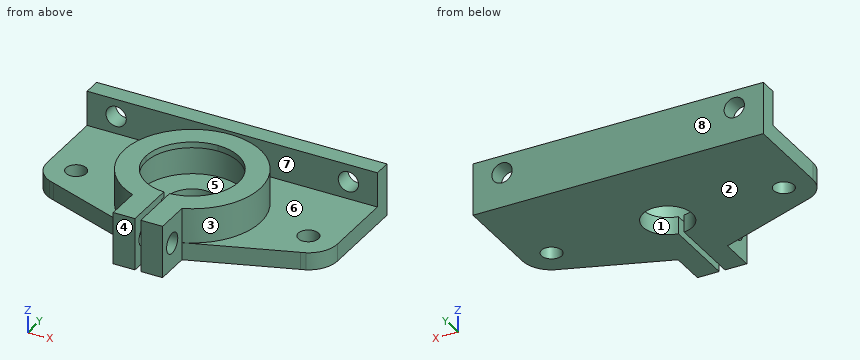
```python
from build123d import *

# Parameters (mm, degrees)
SKETCH1_R                = 3.5
SKETCH1_R_2              = 8.5
BOSS_EXTRUDE1_DEPTH      = 6
SKETCH2_R                = 17.5
BOSS_EXTRUDE2_DEPTH      = 12
SKETCH4_W                = 1.5
SKETCH4_H                = 2
CUT_EXTRUDE1_DEPTH       = 64.087241182
CUT_EXTRUDE1_DEPTH_BACK  = 64.087241182
SKETCH5_R                = 3.5
BOSS_EXTRUDE6_DEPTH      = 50
BOSS_EXTRUDE6_DEPTH_BACK = 50
SKETCH9_W                = 18
SKETCH9_H                = 6
CUT_EXTRUDE10_DEPTH      = 64.087241182
CUT_EXTRUDE10_DEPTH_BACK = 64.087241182
SKETCH10_W               = 2
SKETCH10_H               = 34
SKETCH11_R               = 3.5
CUT_EXTRUDE11_DEPTH      = 80.404030124


with BuildPart() as part:
    # Sketch1 → Boss-Extrude1 (new body)
    with BuildSketch(Plane.XY):
        with BuildLine():
            Line((-42.544589072, -9.670835871), (-8.5, -21.9089023))
            Line((-8.5, -21.9089023), (-8.5, -34))
            Line((-8.5, -34), (8.5, -34))
            Line((8.5, -34), (8.5, -21.9089023))
            Line((8.5, -21.9089023), (42.544589072, -9.670835871))
            Line((42.544589072, -9.670835871), (44.194936835, -9.07758255))
            ThreePointArc((44.194936835, -9.07758255), (48.424647422, -5.38751481), (50, 0))
            Line((50, 0), (50, 25))
            Line((50, 25), (-50, 25))
            Line((-50, 25), (-50, 0))
            ThreePointArc((-50, 0), (-48.424647422, -5.38751481), (-44.194936835, -9.07758255))
            Line((-44.194936835, -9.07758255), (-42.544589072, -9.670835871))
        make_face()
        with Locations((-40, 0)):
            Circle(SKETCH1_R, mode=Mode.SUBTRACT)
        Circle(SKETCH1_R_2, mode=Mode.SUBTRACT)
        with Locations((40, 0)):
            Circle(SKETCH1_R, mode=Mode.SUBTRACT)
    extrude(amount=BOSS_EXTRUDE1_DEPTH)

    # Sketch2 → Boss-Extrude2 (add)
    with BuildSketch(Plane.XY.offset(6)):
        with BuildLine():
            Line((-8.5, -34), (8.5, -34))
            Line((8.5, -34), (8.5, -21.9089023))
            ThreePointArc((8.5, -21.9089023), (0, 23.5), (-8.5, -21.9089023))
            Line((-8.5, -21.9089023), (-8.5, -34))
        make_face()
        Circle(SKETCH2_R, mode=Mode.SUBTRACT)
    extrude(amount=BOSS_EXTRUDE2_DEPTH)

    # Sweep1: sweep along a curve in space
    with BuildLine() as sweep1_path:
        ThreePointArc((17.5, 0, 18), (12.374368671, 12.374368671, 18), (0, 17.5, 18))
        ThreePointArc((0, 17.5, 18), (-12.374368671, 12.374368671, 18), (-17.5, 0, 18))
        ThreePointArc((-17.5, 0, 18), (-12.374368671, -12.374368671, 18), (0, -17.5, 18))
        ThreePointArc((0, -17.5, 18), (12.374368671, -12.374368671, 18), (17.5, 0, 18))
    # Sketch4 → Sweep1 (sweep)
    with BuildSketch(Plane(origin=(0, 0, 0), x_dir=(1, 0, 0), z_dir=(0, 1, 0))):
        with Locations((16.75, -17)):
            Rectangle(SKETCH4_W, SKETCH4_H)
    sweep(path=sweep1_path.line)

    # Sketch5 → Cut-Extrude1 (cut, two sides: drawn at the far end of the back side and taken through both)
    with BuildSketch(Plane(origin=(0, 0, 0), x_dir=(0, 0, -1), z_dir=(1, 0, 0)).offset(-CUT_EXTRUDE1_DEPTH_BACK)):
        with Locations(Location((-9, -28, 0), (0, 0, 180))):
            Circle(SKETCH5_R)
    extrude(amount=CUT_EXTRUDE1_DEPTH + CUT_EXTRUDE1_DEPTH_BACK, mode=Mode.SUBTRACT)

    # Sketch9 → Boss-Extrude6 (add, two sides: drawn at the far end of the back side and taken through both)
    with BuildSketch(Plane(origin=(0, 0, 0), x_dir=(0, 0, -1), z_dir=(1, 0, 0)).offset(-BOSS_EXTRUDE6_DEPTH_BACK)):
        with Locations((-9, 28)):
            Rectangle(SKETCH9_W, SKETCH9_H)
    extrude(amount=BOSS_EXTRUDE6_DEPTH + BOSS_EXTRUDE6_DEPTH_BACK)

    # Sketch10 → Cut-Extrude10 (cut, two sides: drawn at the far end of the back side and taken through both)
    with BuildSketch(Plane.XY.offset(-CUT_EXTRUDE10_DEPTH_BACK)):
        with Locations((0, -17)):
            Rectangle(SKETCH10_W, SKETCH10_H)
    extrude(amount=CUT_EXTRUDE10_DEPTH + CUT_EXTRUDE10_DEPTH_BACK, mode=Mode.SUBTRACT)

    # Sketch11 → Cut-Extrude11 (cut, through all)
    with BuildSketch(Plane.XZ.offset(-25)):
        with Locations(Location((-40, 12, 0), (0, 0, 270))):
            Circle(SKETCH11_R)
        with Locations(Location((40, 12, 0), (0, 0, 270))):
            Circle(SKETCH11_R)
    extrude(amount=-CUT_EXTRUDE11_DEPTH, mode=Mode.SUBTRACT)


solid = part.part
```
Design review of the part built by this model. Coordinates are the model's own, in mm. Face numbers are marked on the shaded views. A direction names the side the tool comes from. Round coordinates to 2 decimals unless told otherwise and drop trailing zeros. Write each loop counter-clockwise with the first axis right and the second up, starting at its lowest first coordinate (ties: lowest second). Pieces come first, ordered by that corner, then holes. Notation, with made-up numbers: (-32.75, 82) -> (-24.75, 82) arc R9 cw to (-24.75, 90) -> close; hole circle Ø7 at (46, -15). An arc over 180 degrees is marked (long way). Write item = value, one per line. Start each with the question number.
1) Take a section at A-A, the plane y = -28. State the section outline as (x, z) points, plus the area to 3 significant figures.
2) Take a section at D-D, the plane y = -4.5. State the section outline as (x, z) points, plus the area to 3 significant figures.
3) Tool access review of the marked faces 4, 5, 6, 7 and 8: name each direction out of +Z, -Z, +X, -X, +Y, -Y from which nothing blocks a thin tool from reaching the whole face with its end or side.
4) Wall thickness on probe 1 along X at (y, z) = (29.8, 12); probe 2 along X at (y, z) = (-1, 5.25); probe 3 along Y at (x, z) = (6.25, 9): over which ranges is each line inside the solid? List them lowest first. Write a range as from..to.
5) Clearance check with flat-ended pins moving along their axes: pin 1 (14 mm diameter, centred on x = -5.5, y = 0, fed in from +Z); pin 2 (3.5 mm diameter, centred on y = -27.5, z = 13, fed in from +X); pin 3 (5.5 mm diameter, centred on y = -18.5, z = 11.5, fed in from +X); pin 4 (4 mm diameter, centred on y = -28, z = 9, fed in from +X). State where each tip first meets the part, or that it passes through.
6) Take a section at B-B, the plane x = 40. State the section outline as (y, z) points.
7) Take a section at C-C, the plane z = 11.25. State the section outline as (x, y) points.
8) Mouldability with a two-part tool opening along X and no side actions: class the marked faces 1, 2 and 3 as +X half, -X half, draft (parallel to the pull), parting line (faces both ways), or undercut.
Results list:
q1.outline = (-8.5, 0) -> (-1, 0) -> (-1, 5.5) -> (-8.5, 5.5) -> close; (-8.5, 12.5) -> (-1, 12.5) -> (-1, 18) -> (-8.5, 18) -> close; (1, 0) -> (8.5, 0) -> (8.5, 5.5) -> (1, 5.5) -> close; (1, 12.5) -> (8.5, 12.5) -> (8.5, 18) -> (1, 18) -> close
q1.area = 165 mm²
q2.outline = (-48.93, 0) -> (-7.21, 0) -> (-7.21, 6) -> (-16.91, 6) -> (-16.91, 16) -> (-15.35, 16) -> (-15.35, 18) -> (-23.07, 18) -> (-23.07, 6) -> (-48.93, 6) -> close; (7.21, 0) -> (48.93, 0) -> (48.93, 6) -> (23.07, 6) -> (23.07, 18) -> (15.35, 18) -> (15.35, 16) -> (16.91, 16) -> (16.91, 6) -> (7.21, 6) -> close
q2.area = 655 mm²
q3.face_4 = +Z, -Z, +X, -X, -Y
q3.face_5 = none
q3.face_6 = +Z
q3.face_7 = +Z, +X, -X
q3.face_8 = +Z, -Z, +X, -X, +Y
q4.probe_1 = -50..-43.5, -36.5..36.5, 43.5..50
q4.probe_2 = -49.95..-43.35, -36.65..-8.44, 8.44..36.65, 43.35..49.95
q4.probe_3 = -34..-31.5, -24.5..-16.35, 16.35..22.65, 25..31
q5.pin_1 = 6
q5.pin_2 = 8.5
q5.pin_3 = 17.44
q5.pin_4 = through
q6.outline = (-10.59, 0) -> (-3.5, 0) -> (-3.5, 6) -> (-10.59, 6) -> close; (3.5, 0) -> (31, 0) -> (31, 8.5) -> (25, 8.5) -> (25, 6) -> (3.5, 6) -> close; (25, 15.5) -> (31, 15.5) -> (31, 18) -> (25, 18) -> close
q7.outline = (-50, 25) -> (-43.42, 25) -> (-43.42, 31) -> (-50, 31) -> close; (-36.58, 25) -> (36.58, 25) -> (36.58, 31) -> (-36.58, 31) -> close; (-8.5, -34) -> (-1, -34) -> (-1, -30.68) -> (-8.5, -30.68) -> close; (-8.5, -25.32) -> (-1, -25.32) -> (-1, -17.47) arc R17.5 cw (long way) to (1, -17.47) -> (1, -25.32) -> (8.5, -25.32) -> (8.5, -21.91) arc R23.5 ccw (long way) to (-8.5, -21.91) -> close; (1, -34) -> (8.5, -34) -> (8.5, -30.68) -> (1, -30.68) -> close; (43.42, 25) -> (50, 25) -> (50, 31) -> (43.42, 31) -> close
q8.face_1 = undercut
q8.face_2 = draft
q8.face_3 = parting line
